from build123d import *


with BuildPart() as f2:
    # F2: sweep along a path in F1
    with BuildLine(Plane.XZ) as f2_path:
        Line((0, 0.1928703859), (-8.5, 0.1928703859))
        Line((-8.5, 0.1928703859), (-10.310026817, 0.9273105534))
        ThreePointArc((-10.310026817, 0.9273105534), (-11.6870349777, 0), (-10.310026817, -0.9273105534))
        Line((-10.310026817, -0.9273105534), (-8.5, -0.2111324798))
        Line((-8.5, -0.2111324798), (0, -0.2111324798))
    # F0 (on Right) → F2 (sweep)
    with BuildSketch(Plane.YZ):
        with BuildLine():
            Line((-1.4866068747, 0.2), (1.4866068747, 0.2))
            ThreePointArc((1.4866068747, 0.2), (0, 1.4883123163), (-1.4866068747, 0.2))
        make_face()
    sweep(path=f2_path.line, transition=Transition.RIGHT)

    # F3: sweep along a path in F1
    with BuildLine(Plane.XZ) as f3_path:
        add(Plane.XZ * Edge.make_bspline(
            [(0, 0.1928703859), (0.2573332154, 0.260272227), (0.8780881589, 0.4261663517), (1.6328392869, 1.207547598), (2.0620173309, 1.6684386646)],
            knots=[0, 0, 0, 0, 0.4125710277, 1, 1, 1, 1], degree=3))
    # F0 (on Right) → F3 (sweep)
    with BuildSketch(Plane.YZ):
        with BuildLine():
            Line((-1.4866068747, 0.2), (1.4866068747, 0.2))
            ThreePointArc((1.4866068747, 0.2), (0, 1.4883123163), (-1.4866068747, 0.2))
        make_face()
    sweep(path=f3_path.line)


solid = f2.part
The listing builds one solid part. Answer for the finished solid, in the listing's coordinates (mm). A direction names the side the tool comes from. Give positions to 0.01 mm unless a question says otherwise; leave off trailing zeros. Use one line per item in the form item = value.
1) Each of these flat-tipped pins is pushed along its axis until it touches: pin 1 (1.8 mm diameter, centred on x = -10.69, z = 0, fed in from +Y); pin 2 (0.9 mm diameter, centred on x = -6, y = 0.5, fed in from +Z). Where does it stop, or does it pass through?
Verdict:
pin_1 = through
pin_2 = 1.49
2) For faces 5 (the cylindrical face through (-8.931, -0.03, 1.766)), 6 (the flat face through (1.82, -0.02, 2.05)), 7 (the flat face through (-4, 0, -0.218)), determine the directions among +Z, -Z, +X, -X, +Y, -Y from which every point of the face is accessible in a straight line to the end or side of a thin tool.
Verdict:
face_5 = +Z
face_6 = +Z, +X, +Y, -Y
face_7 = +X, +Y, -Y
3) The mould has two halves that part along Z. Classify faces 1 (the cylindrical face through (-4.19, -0.03, -1.506)), 2 (the flat face through (-9.39, -0.02, -0.57)), 3 (the flat face through (-9.416, -0.021, 0.572)), 4 (the flat face through (0, 0, -1)): released by +Z, released by -Z, zero draft, split by the parting line, or undercut.
Verdict:
face_1 = released by -Z
face_2 = undercut
face_3 = undercut
face_4 = zero draft
4) Consider probe 1 along Z at (x, y) = (-3, 0); probe 2 along Z at (x, y) = (-3.25, 0.5); probe 3 along X at (y, z) = (-0.1, 0). Determine where each line is inside the solid, lowest interval first. Write a range as [from, to].
Verdict:
probe_1 = [-1.51, -0.22], [0.2, 1.49]
probe_2 = [-1.42, -0.22], [0.2, 1.4]
probe_3 = [-12.98, -11.69]
